Drawing for the job (mm, zero at the part's lowest x, y, z). A direction names the side the tool comes from. Coordinates: 2 decimals unless noted, no trailing zeros. Write each loop counter-clockwise with the first axis right and the second up, starting at its lowest first coordinate (ties: lowest second). Pieces come first, ordered by that corner, then holes. Notation, with made-up numbers: (18.25, -16.5) - (64.25, -16.5) arc R20 cw to (64.25, -10.5) - close; hole circle Ø4 at (84.25, 76.5). An arc over 180 degrees is marked (long way). Write each question's results on one line, items separated by ' | '.
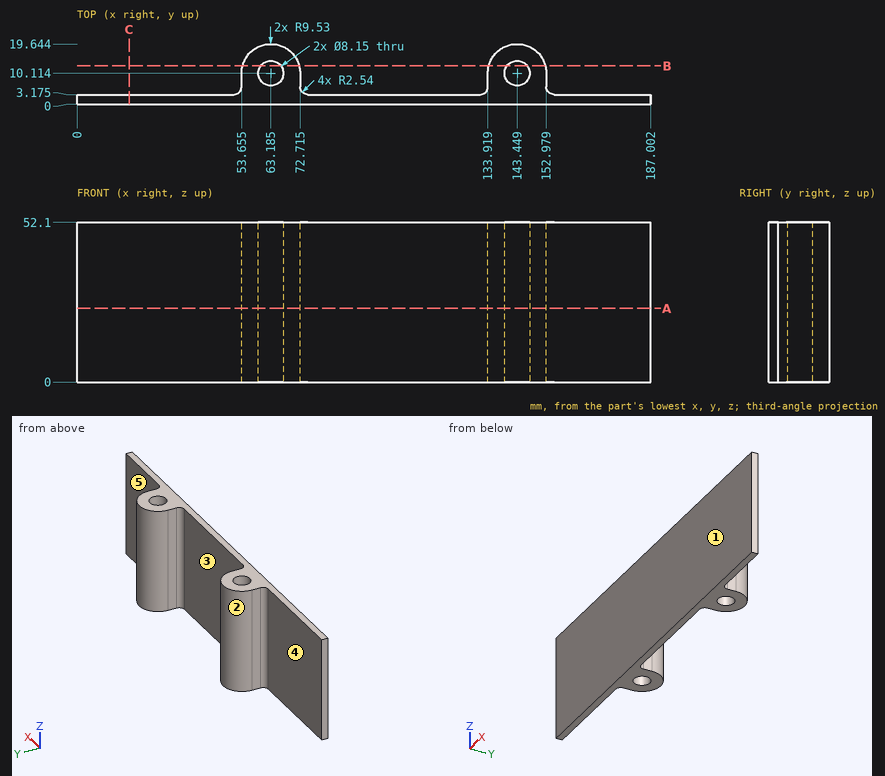
(1) Saw through at C-C on x = 17. Write the cut outline in (y, z) (1 decimal).
Return value:
outline: (0, 0) - (3.2, 0) - (3.2, 52.1) - (0, 52.1) - close
(2) Wall check: line 1 (X direction, y = 9, z = 21) (1 decimal); line 2 (Y direction, x = 11, z = 37) (1 decimal); line 3 (X direction, y = 17, z = 17.5) (1 decimal). Give the ranges that are in metal, low to high. Write a range as from..to.
Return value:
line 1: x = 53.7..59.3, 67.1..72.7, 133.9..139.5, 147.4..153 | line 2: y = 0..3.2 | line 3: x = 56.6..69.8, 136.9..150
(3) Flat gauge pins, fed straight in: P1, Ø1.5, axis at y = 15, z = 16, coming from the -X side; P2, Ø1, axis at x = 36, z = 47, coming from the +Y side (3 decimals); P3, Ø5, axis at x = 78.5, z = 15, coming from the -Y side; P4, Ø2, axis at y = 8.5, z = 30.5, coming from the +X side. Where does each tip first touch, or does it go through?
Return value:
P1: stops at x = 54.6 | P2: stops at y = 3.175 | P3: stops at y = 0 | P4: stops at x = 152.98
(4) Two-plate mould, pull along X, no slides. Class the marked faces 1 and 2: released by +X, released by -X, zero draft, split by the parting line, or undercut.
Return value:
face 1: zero draft | face 2: undercut
(5) 3-axis set-ups, long thin cutter, end or side, ignore diameter. For the marked faces 3, 4 and 5: which of +Z, -Z, +X, -X, +Y, -Y reach the whole face in a straight line?
Return value:
face 3: +Z, -Z, +Y | face 4: +Z, -Z, -X, +Y | face 5: +Z, -Z, +X, +Y
(6) Saw through at A-A on z = 24. Count the separate pieces of the cut face and the enclosed holes in it.
Return value:
separate pieces: 1 | enclosed holes: 2
(7) Saw through at B-B on y = 12.5. Write the cut outline in (x, z) (1 decimal).
Return value:
outline: (54, 0) - (59.9, 0) - (59.9, 52.1) - (54, 52.1) - close; (66.5, 0) - (72.4, 0) - (72.4, 52.1) - (66.5, 52.1) - close; (134.2, 0) - (140.1, 0) - (140.1, 52.1) - (134.2, 52.1) - close; (146.8, 0) - (152.7, 0) - (152.7, 52.1) - (146.8, 52.1) - close
